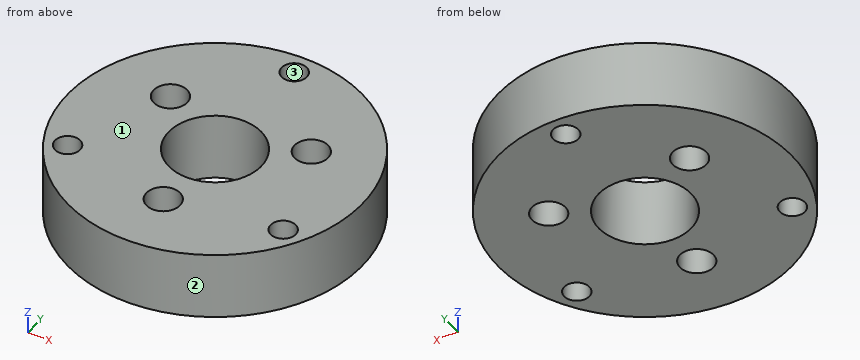
from build123d import *

# Parameters (mm, degrees)
SKETCH_1_R          = 17.5
SKETCH_1_R_2        = 1.5
SKETCH_1_R_3        = 5.5
EXTRUDE_1_DEPTH     = 8
SKETCH_2_R          = 2
CUT_EXTRUDE_1_DEPTH = 19


with BuildPart() as part:
    # 草图1 → 凸台-拉伸1 (new body)
    with BuildSketch(Plane.XY):
        Circle(SKETCH_1_R)
        with Locations((0, 15)):
            Circle(SKETCH_1_R_2, mode=Mode.SUBTRACT)
        with Locations((12.990381057, -7.5)):
            Circle(SKETCH_1_R_2, mode=Mode.SUBTRACT)
        with Locations((-12.990381057, -7.5)):
            Circle(SKETCH_1_R_2, mode=Mode.SUBTRACT)
        Circle(SKETCH_1_R_3, mode=Mode.SUBTRACT)
    extrude(amount=EXTRUDE_1_DEPTH)

    # 草图2 → 切除-拉伸1 (cut)
    with BuildSketch(Plane.XY):
        with Locations((-8.487048957, 4.9)):
            Circle(SKETCH_2_R)
        with Locations((8.487048957, 4.9)):
            Circle(SKETCH_2_R)
        with Locations((0, -9.8)):
            Circle(SKETCH_2_R)
    extrude(amount=CUT_EXTRUDE_1_DEPTH, mode=Mode.SUBTRACT)


solid = part.part
Could you check a few things on this model? Use its own coordinates, in mm. Face numbers are marked on the shaded views. Coordinates: 2 decimals unless noted, no trailing zeros. Order: outer loops, then holes, each group sorted by start corner. A loop starts at its lowest first (then second) coordinate and runs counter-clockwise, first axis right, second up.
Q1. Suppose I cut it at D-D on x = 12.5. Please give me the cut outline in (y, z).
Q2. Please list where these lines run through material, in increasing order: L1, parallel to Y at x = 0, z = 5; L2, parallel to X at y = 6.5, z = 6.5; L3, parallel to X at y = 4.9, z = 2.5.
Q3. Will these pins go through, and if not, where does the flat tip stop? pin 1 (2.5 mm diameter, centred on x = -12.99, y = -7.5, fed in from -Z); pin 2 (1.5 mm diameter, centred on y = -9.5, z = 4.5, fed in from +X); pin 3 (4 mm diameter, centred on y = 3.5, z = 6.5, fed in from -X); pin 4 (1 mm diameter, centred on y = -9, z = 2.5, fed in from -X).
Q4. Suppose I cut it at A-A on z = 6.75. Please give me the cut outline in (x, y).
Q5. Suppose I cut it at B-B on y = 0. Please give me the cut outline in (x, z).
Q6. Suppose I cut it at C-C on x = 0. Please give me the cut outline in (y, z), and give its area (3 significant figures).
Q7. Thinking about a two-plate mould opening in X: for the marked faces 1, 2 and 3, which applies, released by +X, released by -X, zero draft, split by the parting line, or undercut?
Answer:
1. outline: (-12.25, 0) - (-8.92, 0) - (-8.92, 8) - (-12.25, 8) - close; (-6.08, 0) - (12.25, 0) - (12.25, 8) - (-6.08, 8) - close
2. L1: y = -17.5 to -11.8, -7.8 to -5.5, 5.5 to 13.5, 16.5 to 17.5
2. L2: x = -16.25 to -9.69, -7.29 to 7.29, 9.69 to 16.25
2. L3: x = -16.8 to -10.49, -6.49 to -2.5, 2.5 to 6.49, 10.49 to 16.8
3. pin 1: passes through
3. pin 2: stops at x = 15.16
3. pin 3: stops at x = -17.44
3. pin 4: stops at x = -15.3
4. outline: circle Ø35 at (0, 0); hole circle Ø3 at (-12.99, -7.5); hole circle Ø4 at (-8.49, 4.9); hole circle Ø11 at (0, 0); hole circle Ø4 at (0, -9.8); hole circle Ø3 at (0, 15); hole circle Ø4 at (8.49, 4.9); hole circle Ø3 at (12.99, -7.5)
5. outline: (-17.5, 0) - (-5.5, 0) - (-5.5, 8) - (-17.5, 8) - close; (5.5, 0) - (17.5, 0) - (17.5, 8) - (5.5, 8) - close
6. outline: (-17.5, 0) - (-11.8, 0) - (-11.8, 8) - (-17.5, 8) - close; (-7.8, 0) - (-5.5, 0) - (-5.5, 8) - (-7.8, 8) - close; (5.5, 0) - (13.5, 0) - (13.5, 8) - (5.5, 8) - close; (16.5, 0) - (17.5, 0) - (17.5, 8) - (16.5, 8) - close
6. area: 136 mm2
7. face 1: zero draft
7. face 2: split by the parting line
7. face 3: undercut
